Geometry: final body of the model. Coordinates: model frame, mm. A direction names the side the tool comes from. Give positions to 0.01 mm unless a question says otherwise; leave off trailing zeros. Write each loop counter-clockwise with the first axis right and the second up, starting at its lowest first coordinate (ties: lowest second). Pieces come first, ordered by that corner, then holes. Notation, with made-up numbers: (26.25, 9) - (68.25, 9) arc R10 cw to (68.25, 16) - close; hole circle Ø2 at (68, -12.5). An arc over 180 degrees is marked (long way). Use CSV: the item, a comma, the result in double quotes. Start each with the question number.
(1) Line query: probe 1 along Z at (x, y) = (4.75, 0); probe 2 along Z at (x, y) = (15, 0); probe 3 along Y at (x, z) = (7.5, -2.5). Output: solid intervals per line, ascending. Write a range as [from, to].
(2) Section A-A on y = 0. Output: boundary loops of the cut face in (x, z).
(3) Section B-B on z = 0. Output: boundary loops of the cut face in (x, y), and give its area (3 significant figures).
(4) Section C-C on x = 19.5. Output: boundary loops of the cut face in (y, z).
(5) Section D-D on x = 11. Output: boundary loops of the cut face in (y, z).
(6) Reachability of faces 1 (the cylindrical face through (5.976, -14.985, 0.66)), 2 (the flat face through (11, 0, -6.4)), 3 (the flat face through (12, -4, 14)) from +Z, -Z, +X, -X, +Y, -Y: full face, straight path, thin tool, end or side. Return the list, or none.
(7) Draft query along Y for faces 4 (the flat face through (0, 4, -4)), 5 (the cylindrical face through (11, 0, 5)), 6 (the cylindrical face through (10.732, -4.336, -19.524)). Return one class per face: released by +Y, released by -Y, zero draft, split by the parting line, or undercut.
(8) First-contact query: pin 1 Ø9 at (y, z) = (0, 0) entering from -X; pin 2 Ø3.5 at (x, y) = (11.5, 0.5) entering from +Z; pin 3 Ø2 at (x, z) = (3, 10.5) entering from -Y; pin 4 Ø1.3 at (x, z) = (9, -6) entering from +Y. Flat tips, straight axial feed; report the tip coordinate or a pass-through.
from build123d import *

# Parameters (mm, degrees)
CUT_EXTRUDE1_DEPTH = 23
CHAMFER1_SIZE      = 1


with BuildPart() as part:
    # Sketch2 → Revolve1 (revolve)
    with BuildSketch(Plane.XY):
        Polygon((0, 0), (22, 0), (22, 14), (12, 14), (12, 20), (9.5, 20), (7.680148663, 15), (4.319851044, 15), (2.5, 20.000000107), (0, 20.000000107), align=None)
    revolve(axis=Axis((0, 0, 0), (1, 0, 0)))

    # Sketch3 → Cut-Extrude1 (cut, through all)
    with BuildSketch(Plane(origin=(22, 0, 0), x_dir=(0, 0, -1), z_dir=(1, 0, 0))):
        with BuildLine():
            Line((6.4, 1.5), (6.4, -1.5))
            Line((6.4, -1.5), (4.769696007, -1.5))
            ThreePointArc((4.769696007, -1.5), (-5, 0), (4.769696007, 1.5))
            Line((4.769696007, 1.5), (6.4, 1.5))
        make_face()
    extrude(amount=-CUT_EXTRUDE1_DEPTH, mode=Mode.SUBTRACT)

    # Chamfer1
    chamfer1_edges = [part.edges().sort_by_distance(p)[0] for p in [
        (22, -14, 0),
    ]]
    chamfer(chamfer1_edges, length=CHAMFER1_SIZE)


solid = part.part
Check values:
1,probe 1,"z = [-15, -6.4], [5, 15]"
1,probe 2,"z = [-14, -6.4], [5, 14]"
1,probe 3,"y = [-14.79, -4.33], [4.33, 14.79]"
2,outline,"(0, -20) - (2.5, -20) - (4.32, -15) - (7.68, -15) - (9.5, -20) - (12, -20) - (12, -14) - (21, -14) - (22, -13) - (22, -6.4) - (0, -6.4) - close; (0, 5) - (22, 5) - (22, 13) - (21, 14) - (12, 14) - (12, 20) - (9.5, 20) - (7.68, 15) - (4.32, 15) - (2.5, 20) - (0, 20) - close"
3,outline,"(0, -20) - (2.5, -20) - (4.32, -15) - (7.68, -15) - (9.5, -20) - (12, -20) - (12, -14) - (21, -14) - (22, -13) - (22, -5) - (0, -5) - close; (0, 5) - (22, 5) - (22, 13) - (21, 14) - (12, 14) - (12, 20) - (9.5, 20) - (7.68, 15) - (4.32, 15) - (2.5, 20) - (0, 20) - close"
3,area,"487 mm²"
4,outline,"circle Ø28 at (0, 0); hole (-1.5, -6.4) - (1.5, -6.4) - (1.5, -4.77) arc R5 ccw (long way) to (-1.5, -4.77) - close"
5,outline,"circle Ø40 at (0, 0); hole (-1.5, -6.4) - (1.5, -6.4) - (1.5, -4.77) arc R5 ccw (long way) to (-1.5, -4.77) - close"
6,face 1,"none"
6,face 2,"+X, -X"
6,face 3,"+X"
7,face 4,"zero draft"
7,face 5,"undercut"
7,face 6,"split by the parting line"
8,pin 1,"passes through"
8,pin 2,"stops at z = 20"
8,pin 3,"stops at y = -17.53"
8,pin 4,"stops at y = 19.2"
